```python
from build123d import *

# Parameters (mm, degrees)
F0_W     = 152.4
F0_H     = 147.32
F1_DEPTH = 88.9
F2_W     = 62.077993
F2_H     = 60.928402
F2_W_2   = 28.548219
F2_H_2   = 16.669087
F3_DEPTH = 5.08


with BuildPart() as f1:
    # F0 (on Top) → F1 (new body)
    with BuildSketch(Plane.XY):
        with Locations((76.2, 73.66)):
            Rectangle(F0_W, F0_H)
    extrude(amount=F1_DEPTH)

    # F2 (on face) → F3 (cut)
    with BuildSketch(Plane.XZ):
        with Locations((45.143026, 45.622946)):
            Rectangle(F2_W, F2_H)
        with Locations((118.237953, 63.34583)):
            Rectangle(F2_W_2, F2_H_2)
    extrude(amount=-F3_DEPTH, mode=Mode.SUBTRACT)


solid = f1.part
```
Could you check a few things on this model? Use its own coordinates, in mm. A direction names the side the tool comes from. Round coordinates to 2 decimals unless told otherwise and drop trailing zeros. Loops run counter-clockwise (first coordinate to the right, second up) from the corner with the lowest first, then second, coordinate; pieces in that order, holes last. Notation, with made-up numbers: (49.5, 48) -> (74.5, 48) arc R23 ccw to (74.5, 82) -> close; hole circle Ø9 at (11, -13). An arc over 180 degrees is marked (long way). One line per question, with ' | ' between items.
(1) For faces 1 (the face through (76.182, 3, 45)), 2 (the face through (152.4, 73, 44)), which set-ups out of +Z, -Z, +X, -X, +Y, -Y let a thin tool reach every point of the face, with its end or its side?
Model answer:
face 1: -Y | face 2: +Z, -Z, +X, +Y, -Y
(2) For pin 1 Ø1 at (y, z) = (101, 38) entering from -X, with a flat end and sliding along its axis, tell me the tip position at first contact or that it passes through.
Model answer:
pin 1: stops at x = 0
(3) Thinking about a two-plate mould opening in Z: for faces 3 (the face through (132.512, 3, 63)), 4 (the face through (75, 75, 88.9)), 5 (the face through (92, 0, 44)), 6 (the face through (75, 75, 0)), which applies, released by +Z, released by -Z, zero draft, split by the parting line, or undercut?
Model answer:
face 3: undercut | face 4: released by +Z | face 5: zero draft | face 6: released by -Z
(4) If I drill on probe 1 along Y at (x, z) = (51, 74), over which ranges is the centre line in solid material (lowest first)?
Model answer:
probe 1: y = 5.08 to 147.32
(5) If we section it at A-A on x = 72: List the corners of the cut face in (y, z) for me.
Model answer:
outline: (0, 0) -> (147.32, 0) -> (147.32, 88.9) -> (0, 88.9) -> (0, 76.09) -> (5.08, 76.09) -> (5.08, 15.16) -> (0, 15.16) -> close
